The model under review builds one solid part; all positions refer to its coordinate system, in mm. A direction names the side the tool comes from. Round coordinates to 2 decimals unless told otherwise and drop trailing zeros. Write each loop counter-clockwise with the first axis right and the second up, starting at its lowest first coordinate (ties: lowest second). Pieces come first, ordered by that corner, then holes. Notation, with made-up numbers: (28, 58) -> (49, 58) arc R34 ccw to (49, 89) -> close; hole circle Ø11 at (17.25, 78.25). An arc over 180 degrees is marked (long way). Answer as a JSON object with one key per item and string values. Group by question number.
1) We need section D-D, the plane x = -55.5. Write out the cut boundary in (y, z) (3 decimals), then the cut area to 3 significant figures.
2) To check wall thickness, follow probe 1 along X at (y, z) = (-2.75, 5.5); probe 2 along Y at (x, z) = (-57.15, 2) (3 decimals); probe 3 along Y at (x, z) = (-10.5, 6). State the ranges of each line that lie inside material, in increasing order. Write a range as [from, to].
3) Machinability: for faces 4 (the flat face through (34, 9.525, 3)), 5 (the flat face through (34, -9.525, 3)), 6 (the cylindrical face through (-53.63, -1.46, 3.13)), 7 (the flat face through (-34, -9.525, 3)), 8 (the cylindrical face through (0.1, -12.7, 3.1)), which of the approach directions +Z, -Z, +X, -X, +Y, -Y give a long, thin tool a straight path to every point of the face, cutting with its end or side? Answer none if there is none.
4) Mouldability with a two-part tool opening along Y and no side actions: class faces 1 (the cylindrical face through (-1.38, -6.2, 3.13)), 2 (the flat face through (-34, 9.525, 3)), 3 (the cylindrical face through (-66.673, -0.209, 3.131)) as pulls with the +Y half, pulls with the -Y half, needs draft (parallel to the pull), parting line crosses it, or undercut.
5) We need section A-A, the plane x = 0. Write out the cut boundary in (y, z), then the cut area to 3 significant figures.
6) We need section B-B, the plane y = 0. Write out the cut boundary in (x, z) (3 decimals).
7) We need section C-C, the plane z = 1.75. Write out the cut boundary in (x, y) (3 decimals).
8) Insertion check: pin 1 Ø10 at (x, y) = (39, 5) entering from -Z; pin 2 Ø1.5 at (x, z) = (-28, 3) entering from +Y (3 decimals); pin 3 Ø3 at (x, z) = (-42, 3.5) entering from -Y (3 decimals); pin 4 Ø1.5 at (y, z) = (7, 4) entering from -X. Each pin has a flat end and moves straight along its axis. Give the tip position at first contact, or say it passes through.
from build123d import *

# Parameters (mm, degrees)
SKETCH1_R           = 3.81
SKETCH1_R_2         = 6.35
BOSS_EXTRUDE1_DEPTH = 6.35


with BuildPart() as part:
    # Sketch1 → Boss-Extrude1 (new body)
    with BuildSketch(Plane.XY):
        with BuildLine():
            Line((-57.15, 9.525), (-10.530283709, 9.525))
            ThreePointArc((-10.530283709, 9.525), (-8.697196605, 9.795337866), (-7.02018914, 10.583333333))
            ThreePointArc((-7.02018914, 10.583333333), (0, 12.7), (7.02018914, 10.583333333))
            ThreePointArc((7.02018914, 10.583333333), (8.697196605, 9.795337866), (10.530283709, 9.525))
            Line((10.530283709, 9.525), (57.15, 9.525))
            ThreePointArc((57.15, 9.525), (66.675, 0), (57.15, -9.525))
            Line((57.15, -9.525), (10.530283709, -9.525))
            ThreePointArc((10.530283709, -9.525), (8.697196605, -9.795337866), (7.02018914, -10.583333333))
            ThreePointArc((7.02018914, -10.583333333), (0, -12.7), (-7.02018914, -10.583333333))
            ThreePointArc((-7.02018914, -10.583333333), (-8.697196605, -9.795337866), (-10.530283709, -9.525))
            Line((-10.530283709, -9.525), (-57.15, -9.525))
            ThreePointArc((-57.15, -9.525), (-66.675, 0), (-57.15, 9.525))
        make_face()
        with Locations((-57.15, 0)):
            Circle(SKETCH1_R, mode=Mode.SUBTRACT)
        with Locations((57.15, 0)):
            Circle(SKETCH1_R, mode=Mode.SUBTRACT)
        Circle(SKETCH1_R_2, mode=Mode.SUBTRACT)
    extrude(amount=BOSS_EXTRUDE1_DEPTH)


solid = part.part
Here are the results:
{
 "1": {"outline": "(-9.525, 0) -> (-3.434, 0) -> (-3.434, 6.35) -> (-9.525, 6.35) -> close; (3.434, 0) -> (9.525, 0) -> (9.525, 6.35) -> (3.434, 6.35) -> close", "area": "77.4 mm^2"},
 "2": {"probe 1": "x = [-66.27, -59.79], [-54.51, -5.72], [5.72, 54.51], [59.79, 66.27]", "probe 2": "y = [-9.525, -3.81], [3.81, 9.525]", "probe 3": "y = [-9.53, 9.53]"},
 "3": {"face 4": "+Z, -Z, +X, +Y", "face 5": "+Z, -Z, +X, -Y", "face 6": "+Z, -Z", "face 7": "+Z, -Z, -X, -Y", "face 8": "+Z, -Z, -Y"},
 "4": {"face 1": "undercut", "face 2": "pulls with the +Y half", "face 3": "parting line crosses it"},
 "5": {"outline": "(-12.7, 0) -> (-6.35, 0) -> (-6.35, 6.35) -> (-12.7, 6.35) -> close; (6.35, 0) -> (12.7, 0) -> (12.7, 6.35) -> (6.35, 6.35) -> close", "area": "80.6 mm^2"},
 "6": {"outline": "(-66.675, 0) -> (-60.96, 0) -> (-60.96, 6.35) -> (-66.675, 6.35) -> close; (-53.34, 0) -> (-6.35, 0) -> (-6.35, 6.35) -> (-53.34, 6.35) -> close; (6.35, 0) -> (53.34, 0) -> (53.34, 6.35) -> (6.35, 6.35) -> close; (60.96, 0) -> (66.675, 0) -> (66.675, 6.35) -> (60.96, 6.35) -> close"},
 "7": {"outline": "(-57.15, -9.525) -> (-10.53, -9.525) arc R6.35 cw to (-7.02, -10.583) arc R12.7 ccw to (7.02, -10.583) arc R6.35 cw to (10.53, -9.525) -> (57.15, -9.525) arc R9.525 ccw to (57.15, 9.525) -> (10.53, 9.525) arc R6.35 cw to (7.02, 10.583) arc R12.7 ccw to (-7.02, 10.583) arc R6.35 cw to (-10.53, 9.525) -> (-57.15, 9.525) arc R9.525 ccw to start; hole circle Ø7.62 at (-57.15, 0); hole circle Ø12.7 at (0, 0); hole circle Ø7.62 at (57.15, 0)"},
 "8": {"pin 1": "stops at z = 0", "pin 2": "stops at y = 9.525", "pin 3": "stops at y = -9.525", "pin 4": "stops at x = -64.34"}
}
